Design review of the part built by this model. Coordinates are the model's own, in mm. Face numbers are marked on the shaded views. A direction names the side the tool comes from. Coordinates: 2 decimals unless noted, no trailing zeros. Loops run counter-clockwise (first coordinate to the right, second up) from the corner with the lowest first, then second, coordinate; pieces in that order, holes last.
Q1. For P1, Ø8.5, axis at x = -91.5, z = 43.5, coming from the -Y side; P2, Ø8, axis at x = -84, y = 45.5, coming from the +Z side; P3, Ø4, axis at y = 0.5, z = 42, coming from the +X side, all flat-tipped, find the tip position at first contact; note any pin that passes through.
Q2. Add section C-C on y = 37. Give the boundary of the cut face in (x, z).
Q3. Add section A-A on y = 24. Give the boundary of the cut face in (x, z).
Q4. Add section B-B on x = 43.5. Give the boundary of the cut face in (y, z), and give its area (3 significant figures).
Q5. Draft analysis for pull direction X (two halves, no side actions). For the marked faces 1, 2 and 3, state which applies: released by +X, released by -X, zero draft, split by the parting line, or undercut.
Q6. Machinability: for the marked faces 4, 5 and 6, which of the approach directions +Z, -Z, +X, -X, +Y, -Y give a long, thin tool a straight path to every point of the face, cutting with its end or side? Answer none if there is none.
Q7. Wall thickness on probe 1 along Z at (x, y) = (-12, 18.5); probe 2 along Z at (x, y) = (-86, -17); probe 3 along Y at (x, z) = (-83, 38.5): over which ranges is each line inside the solid? List them lowest first.
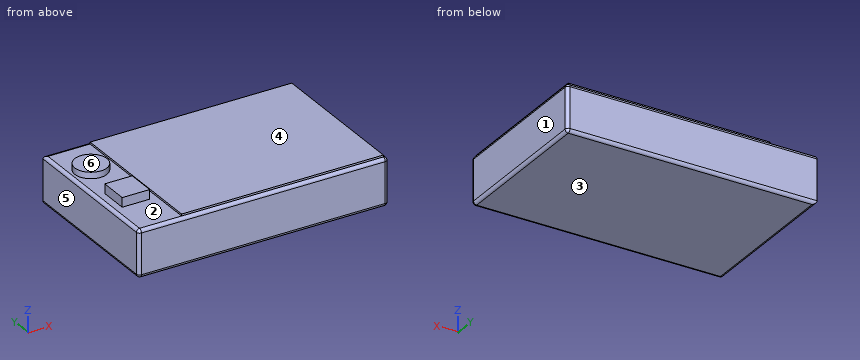
```python
from build123d import *

# Parameters (mm, degrees)
F0_W     = 203.2
F0_H     = 127
F1_DEPTH = 38.1
F2_R     = 2.54
F3_R     = 13.086022
F4_DEPTH = 5.08
F5_W     = 22.316434
F5_H     = 23.267692
F6_DEPTH = 7.62
F7_W     = 163.913434
F7_H     = 121.92
F8_DEPTH = 1.524


with BuildPart() as f1:
    # F0 (on Top) → F1 (new body)
    with BuildSketch(Plane.XY):
        with Locations((-6.043922, 12.433724)):
            Rectangle(F0_W, F0_H)
    extrude(amount=F1_DEPTH)

    # F2
    f2_edges = [f1.edges().sort_by_distance(p)[0] for p in [
        (-6.043922, -51.066276, 0),
        (-6.043922, -51.066276, 38.1),
        (-107.643922, -51.066276, 19.05),
        (95.556078, -51.066276, 19.05),
        (95.556078, 12.433724, 38.1),
        (95.556078, 12.433724, 0),
        (95.556078, 75.933724, 19.05),
        (-6.043922, 75.933724, 38.1),
        (-107.643922, 12.433724, 38.1),
        (-6.043922, 75.933724, 0),
        (-107.643922, 12.433724, 0),
    ]]
    fillet(f2_edges, radius=F2_R)

    # F3 (on face) → F4 (join)
    with BuildSketch(Plane.XY.offset(38.1)):
        with Locations((-89.747429, 41.45414)):
            Circle(F3_R)
    extrude(amount=F4_DEPTH)

    # F5 (on face) → F6 (join)
    with BuildSketch(Plane.XY.offset(38.1)):
        with Locations((-88.330593, -4.60028)):
            Rectangle(F5_W, F5_H)
    extrude(amount=F6_DEPTH)

    # F7 (on face) → F8 (join)
    with BuildSketch(Plane.XY.offset(38.1)):
        with Locations((11.059361, 12.433724)):
            Rectangle(F7_W, F7_H)
    extrude(amount=F8_DEPTH)


solid = f1.part
```
Entries:
1. P1: stops at y = -16.23
1. P2: stops at z = 43.18
1. P3: stops at x = -77.17
2. outline: (-107.64, 2.54) arc R2.54 ccw to (-105.1, 0) - (93.02, 0) arc R2.54 ccw to (95.56, 2.54) - (95.56, 35.56) arc R2.54 ccw to (93.02, 38.1) - (93.02, 39.62) - (-70.9, 39.62) - (-70.9, 38.1) - (-77.44, 38.1) - (-77.44, 43.18) - (-102.05, 43.18) - (-102.05, 38.1) - (-105.1, 38.1) arc R2.54 ccw to (-107.64, 35.56) - close
3. outline: (-107.64, 2.54) arc R2.54 ccw to (-105.1, 0) - (93.02, 0) arc R2.54 ccw to (95.56, 2.54) - (95.56, 35.56) arc R2.54 ccw to (93.02, 38.1) - (93.02, 39.62) - (-70.9, 39.62) - (-70.9, 38.1) - (-105.1, 38.1) arc R2.54 ccw to (-107.64, 35.56) - close
4. outline: (-51.07, 2.54) arc R2.54 ccw to (-48.53, 0) - (73.39, 0) arc R2.54 ccw to (75.93, 2.54) - (75.93, 35.56) arc R2.54 ccw to (73.39, 38.1) - (73.39, 39.62) - (-48.53, 39.62) - (-48.53, 38.1) arc R2.54 ccw to (-51.07, 35.56) - close
4. area: 5,020 mm2
5. face 1: released by +X
5. face 2: undercut
5. face 3: zero draft
6. face 4: +Z, +X, +Y, -Y
6. face 5: +Z, -Z, -X, +Y, -Y
6. face 6: +Z, +X, -X, +Y
7. probe 1: z = 0 to 39.62
7. probe 2: z = 0 to 38.1
7. probe 3: y = -16.23 to 7.03, 30.24 to 52.67
